The drawing under review shows one solid part. Ordinate dimensions are in mm from its lowest x, y, z. Give positions to 0.01 mm unless a question says otherwise; leave off trailing zeros. Order: outer loops, then holes, each group sorted by start corner. A loop starts at its lowest first (then second) coordinate and runs counter-clockwise, first axis right, second up. Notation, with made-up numbers: (57.5, -18) -> (83.5, -18) arc R33 ccw to (83.5, 10) -> close; hole circle Ø2 at (-37, 69.25). An arc over 180 degrees is marked (long way). One line per item, written item: value.
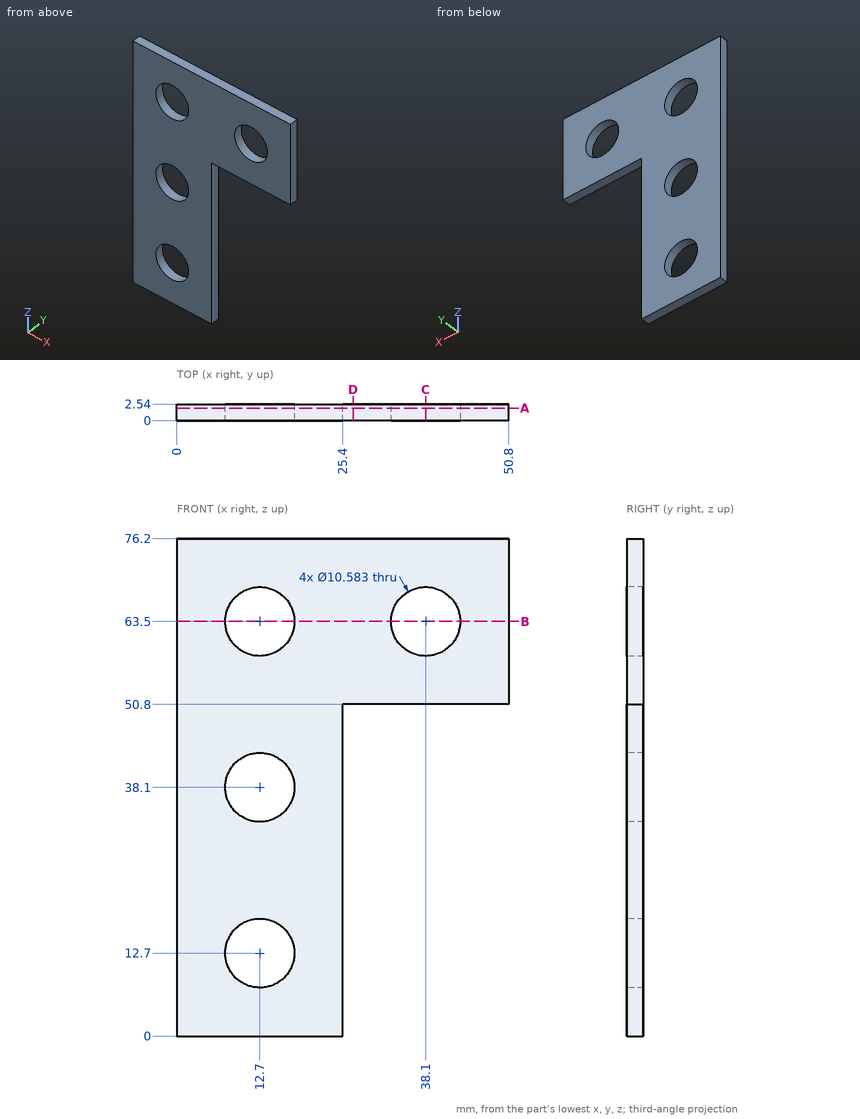
Item 1: Add section C-C on x = 38.1. Give the boundary of the cut face in (y, z).
Returned:
outline: (0, 50.8) -> (2.54, 50.8) -> (2.54, 58.21) -> (0, 58.21) -> close; (0, 68.79) -> (2.54, 68.79) -> (2.54, 76.2) -> (0, 76.2) -> close
Item 2: Add section A-A on y = 1.9. Give the boundary of the cut face in (x, z).
Returned:
outline: (0, 0) -> (25.4, 0) -> (25.4, 50.8) -> (50.8, 50.8) -> (50.8, 76.2) -> (0, 76.2) -> close; hole circle Ø10.58 at (12.7, 12.7); hole circle Ø10.58 at (12.7, 38.1); hole circle Ø10.58 at (12.7, 63.5); hole circle Ø10.58 at (38.1, 63.5)
Item 3: Add section D-D on x = 27. Give the boundary of the cut face in (y, z).
Returned:
outline: (0, 50.8) -> (2.54, 50.8) -> (2.54, 76.2) -> (0, 76.2) -> close
Item 4: Clearance check with a flat-ended pin moving along its axis: P1, Ø0.8, axis at y = 0.5, z = 31.5, coming from the +X side. State where the tip first meets the part, or that it passes through.
Returned:
P1: x = 25.4
Item 5: Add section B-B on z = 63.5. Give the boundary of the cut face in (x, y).
Returned:
outline: (0, 0) -> (7.41, 0) -> (7.41, 2.54) -> (0, 2.54) -> close; (17.99, 0) -> (32.81, 0) -> (32.81, 2.54) -> (17.99, 2.54) -> close; (43.39, 0) -> (50.8, 0) -> (50.8, 2.54) -> (43.39, 2.54) -> close
Item 6: To check wall thickness, follow line 1 along Z through (x, y) = (12.7, 2.05); line 2 along Z through (x, y) = (38.1, 2); line 3 along X through (y, z) = (0.9, 64.5). State the ranges of each line that lie inside material, in increasing order. Write a range as from..to.
Returned:
line 1: 0..7.41, 17.99..32.81, 43.39..58.21, 68.79..76.2
line 2: 50.8..58.21, 68.79..76.2
line 3: 0..7.5, 17.9..32.9, 43.3..50.8
